The model under review builds one solid part; all positions refer to its coordinate system, in mm. Round coordinates to 2 decimals unless told otherwise and drop trailing zeros. Write each loop counter-clockwise with the first axis right and the second up, starting at its lowest first coordinate (ties: lowest second). Pieces come first, ordered by that corner, then holes. Notation, with made-up numbers: M -31,84.25 L -26,84.25 A18 cw -26,116.25 Z; hole C -10.5,11 d1. An arc over 180 degrees is marked long. One line per item, written item: value. Start each with the question number.
1) Take a section at D-D, the plane z = -19. Write out the cut boundary in (x, y).
2) Wall thickness on probe 1 along Z at (x, y) = (0, 1.35); probe 2 along Z at (x, y) = (44, 0.5): over which ranges is each line inside the solid? List them lowest first.
3) Take a section at C-C, the plane z = 0. Write out the cut boundary in (x, y).
4) Take a section at B-B, the plane y = 1.3. State how many separate pieces and enclosed holes the cut face has, and give its area (3 significant figures).
5) Take a section at A-A, the plane x = 0. Write out the cut boundary in (y, z).
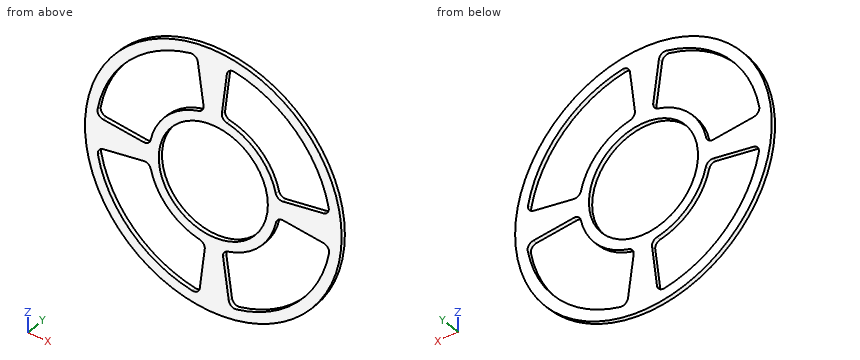
from build123d import *

# Parameters (mm, degrees)
SKETCH1_R           = 60
SKETCH1_R_2         = 25.5
BOSS_EXTRUDE1_DEPTH = 2
CUT_EXTRUDE1_DEPTH  = 2
CIRPATTERN1_COUNT   = 4


with BuildPart() as part:
    # Sketch1 → Boss-Extrude1 (new body)
    with BuildSketch(Plane(origin=(0, 0, 0), x_dir=(1, 0, 0), z_dir=(0, 1, 0))):
        Circle(SKETCH1_R)
        Circle(SKETCH1_R_2, mode=Mode.SUBTRACT)
    extrude(amount=BOSS_EXTRUDE1_DEPTH)

    # Sketch2 → Cut-Extrude1 (cut)
    with BuildSketch(Plane(origin=(0, 2, 0), x_dir=(1, 0, 0), z_dir=(0, 1, 0))):
        with BuildLine():
            Line((-32.618394997, -4.005035307), (-51.526434877, -6.326650681))
            ThreePointArc((-51.526434877, -6.326650681), (-53.577175122, -7.526295601), (-54.112413011, -9.841075048))
            ThreePointArc((-54.112413011, -9.841075048), (-39.228774703, -38.550009536), (-10.78396803, -53.932420987))
            ThreePointArc((-10.78396803, -53.932420987), (-8.460199946, -53.437663089), (-7.224947385, -51.408171873))
            Line((-7.224947385, -51.408171873), (-4.573694808, -32.543529554))
            ThreePointArc((-4.573694808, -32.543529554), (-5.068923242, -30.431452905), (-6.858635467, -29.205463864))
            ThreePointArc((-6.858635467, -29.205463864), (-21.397513475, -21.027277929), (-29.320715424, -6.347885238))
            ThreePointArc((-29.320715424, -6.347885238), (-30.515282955, -4.537049136), (-32.618394997, -4.005035307))
        make_face()
    cut_extrude1 = extrude(amount=-CUT_EXTRUDE1_DEPTH, mode=Mode.SUBTRACT)

    # CirPattern1: Cut-Extrude1 ×4 about axis
    cirpattern1_axis = Axis((0, 0, 0), (0, 1, 0))
    for i in range(1, CIRPATTERN1_COUNT):
        add(cut_extrude1.rotate(cirpattern1_axis, i * 360 / CIRPATTERN1_COUNT), mode=Mode.SUBTRACT)


solid = part.part
Checked values:
1. outline: M -56.91,0 L -51.61,0 L -51.61,2 L -56.91,2 Z; M -23.22,0 L -17.01,0 L -17.01,2 L -23.22,2 Z; M 17.01,0 L 23.22,0 L 23.22,2 L 17.01,2 Z; M 51.61,0 L 56.91,0 L 56.91,2 L 51.61,2 Z
2. probe 1: z = -60 to -25.5, 25.5 to 60
2. probe 2: z = -40.79 to -33, -5.4 to 6.18, 33 to 40.79
3. outline: M -60,0 L -25.5,0 L -25.5,2 L -60,2 Z; M 25.5,0 L 60,0 L 60,2 L 25.5,2 Z
4. separate pieces: 1
4. enclosed holes: 5
4. area: 3,730 mm2
5. outline: M 0,-60 L 2,-60 L 2,-25.5 L 0,-25.5 Z; M 0,25.5 L 2,25.5 L 2,60 L 0,60 Z
